Source: CAD feature listing. Evaluate the final solid. Frame: model axes, mm. A direction names the side the tool comes from. Coordinates: 2 decimals unless noted, no trailing zeros. Loops run counter-clockwise (first coordinate to the right, second up) from the corner with the lowest first, then second, coordinate; pieces in that order, holes last. Notation, with made-up numbers: (47.5, 17.5) - (81.5, 17.5) arc R18 cw to (81.5, 26.5) - close; hole circle Ø9 at (2.5, 28.5). An arc over 180 degrees is marked (long way). Write item = value, one per line. Start each with the question number.
from build123d import *

# Parameters (mm, degrees)
SKETCH1_W           = 3.302
SKETCH1_H           = 3.302
BOSS_EXTRUDE1_DEPTH = 31.5595
SKETCH2_R           = 1.27
CUT_EXTRUDE1_DEPTH  = 3.175


with BuildPart() as part:
    # Sketch1 → Boss-Extrude1 (new body, symmetric)
    with BuildSketch(Plane(origin=(0, 0, 0), x_dir=(0, 0, -1), z_dir=(1, 0, 0))):
        Rectangle(SKETCH1_W, SKETCH1_H)
    extrude(amount=BOSS_EXTRUDE1_DEPTH, both=True)

    # Sketch2 → Cut-Extrude1 (cut)
    with BuildSketch(Plane(origin=(31.5595, 0, 0), x_dir=(0, 0, -1), z_dir=(1, 0, 0))):
        Circle(SKETCH2_R)
    cut_extrude1 = extrude(amount=-CUT_EXTRUDE1_DEPTH, mode=Mode.SUBTRACT)

    # Mirror1: Cut-Extrude1 across plane
    add(cut_extrude1.mirror(Plane(origin=(0, 0, 0), x_dir=(0, 0, 1), z_dir=(1, 0, 0))), mode=Mode.SUBTRACT)


solid = part.part
Item 1: First-contact query: pin 1 (1.5 mm diameter, centred on y = 0, z = 0, fed in from -X). Flat tip, straight axial feed; report the tip coordinate or a pass-through.
Item 2: Material intervals for L1, parallel to Y at x = -29.35, z = 0; L2, parallel to X at y = -0.4, z = -0.65; L3, parallel to Y at x = 28.5, z = -0.75, sorted ascending. Write a range as [from, to].
Item 3: Cut plane B-B (y = -0.55). Return the cut outline in (x, z), then the cut area to 3 significant figures.
Item 4: Draft query along Z for faces 1 (the flat face through (0, 0, 1.651)), 2 (the flat face through (-28.384, 0, 0)), 3 (the flat face through (0, 1.651, 0)), 4 (the flat face through (0, 0, -1.651)). Return one class per face: released by +Z, released by -Z, zero draft, split by the parting line, or undercut.
Item 5: Reachability of faces 5 (the flat face through (0, -1.651, 0)), 6 (the cylindrical face through (-29.99, 1.26, 0.17)), 7 (the flat face through (28.384, 0, 0)) from +Z, -Z, +X, -X, +Y, -Y: full face, straight path, thin tool, end or side. Return the list, or none.
Item 6: Cut plane A-A (z = 0). Return the cut outline in (x, y), then the cut area to 3 significant figures.
Responses:
q1.pin_1 = -28.38
q2.L1 = [-1.65, -1.27], [1.27, 1.65]
q2.L2 = [-28.38, 28.38]
q2.L3 = [-1.65, -1.02], [1.02, 1.65]
q3.outline = (-31.56, -1.65) - (31.56, -1.65) - (31.56, -1.14) - (28.38, -1.14) - (28.38, 1.14) - (31.56, 1.14) - (31.56, 1.65) - (-31.56, 1.65) - (-31.56, 1.14) - (-28.38, 1.14) - (-28.38, -1.14) - (-31.56, -1.14) - close
q3.area = 194 mm2
q4.face_1 = released by +Z
q4.face_2 = undercut
q4.face_3 = zero draft
q4.face_4 = released by -Z
q5.face_5 = +Z, -Z, +X, -X, -Y
q5.face_6 = -X
q5.face_7 = +X
q6.outline = (-31.56, -1.65) - (31.56, -1.65) - (31.56, -1.27) - (28.38, -1.27) - (28.38, 1.27) - (31.56, 1.27) - (31.56, 1.65) - (-31.56, 1.65) - (-31.56, 1.27) - (-28.38, 1.27) - (-28.38, -1.27) - (-31.56, -1.27) - close
q6.area = 192 mm2
